Read the model definition and answer for the solid it produces. Units are mm, in the model's axes. Round coordinates to 2 decimals unless told otherwise and drop trailing zeros. Order: outer loops, then holes, each group sorted by start corner. A loop starts at its lowest first (then second) coordinate and runs counter-clockwise, first axis right, second up. Notation, with made-up numbers: (-39.75, 23.5) - (-29.75, 23.5) arc R20 cw to (-29.75, 57.5) - close; hole circle Ø8 at (18, -18). An arc over 180 degrees is marked (long way). Answer as a JSON object with one key per item and string values. Group by question number.
Q1. A cutting plane is placed at D-D on x = 41. Determine the outline of the cut face in (y, z) (3 decimals).
Q2. Given pin 1 Ø0.5 at (y, z) = (1, 1) entering from +X, flat-ended and moving along its own axis, determine where the tip first touches the part or whether it passes through.
Q3. A cutting plane is placed at C-C on x = 20.5. Determine the outline of the cut face in (y, z) (3 decimals), and give its area (3 significant figures).
Q4. Consider line 1 (X direction, y = 0.5, z = 1.8); line 2 (X direction, y = -5.5, z = 3.05); line 3 (Y direction, x = 21, z = 1.35). Determine where each line is inside the solid, lowest interval first.
Q5. A cutting plane is placed at B-B on z = 1.3. Count the separate pieces of the cut face and the enclosed holes in it, and give its area (3 significant figures).
Q6. A cutting plane is placed at A-A on y = -54.5. Determine the outline of the cut face in (x, z) (3 decimals).
Q7. The mould has two halves that part along Y. Classify faces 1 (the cylindrical face through (59.551, -59.674, 1.565)), 2 (the cylindrical face through (82.194, -74.995, 1.565)), 3 (the cylindrical face through (-24.02, 11.11, 1.57)): pulls with the +Y half, pulls with the -Y half, needs draft (parallel to the pull), parting line crosses it, or undercut.
```python
from build123d import *

# Parameters (mm, degrees)
SKETCH1_R           = 5.275384615
SKETCH1_R_2         = 3.2639
BOSS_EXTRUDE1_DEPTH = 3.175


with BuildPart() as part:
    # Sketch1 → Boss-Extrude1 (new body)
    with BuildSketch(Plane.XY):
        with BuildLine():
            Line((-14.2875, 1.5875), (-14.2875, 0))
            ThreePointArc((-14.2875, 0), (0, -14.2875), (14.2875, 0))
            Line((14.2875, 0), (14.2875, 1.5875))
            ThreePointArc((14.2875, 1.5875), (20.740075347, 10.603365557), (31.355391181, 7.403892149))
            Line((31.355391181, 7.403892149), (82.572922645, -59.016709578))
            ThreePointArc((82.572922645, -59.016709578), (82.033512438, -75.180341372), (66.05971387, -77.708525595))
            Line((66.05971387, -77.708525595), (-16.947053899, -28.708644524))
            ThreePointArc((-16.947053899, -28.708644524), (-28.951349844, -16.529012325), (-33.3375, 0))
            Line((-33.3375, 0), (-33.3375, 1.5875))
            ThreePointArc((-33.3375, 1.5875), (-23.8125, 11.1125), (-14.2875, 1.5875))
        make_face()
        with Locations((-23.8125, 0)):
            Circle(SKETCH1_R, mode=Mode.SUBTRACT)
        with Locations((23.8125, 0)):
            Circle(SKETCH1_R, mode=Mode.SUBTRACT)
        with Locations((72.515734403, -66.77189911)):
            Circle(SKETCH1_R_2, mode=Mode.SUBTRACT)
        with Locations((60.259023314, -56.487297355)):
            Circle(SKETCH1_R_2, mode=Mode.SUBTRACT)
    extrude(amount=BOSS_EXTRUDE1_DEPTH)


solid = part.part
```
Result set:
{
 "1": {"outline": "(-62.915, 0) - (-5.104, 0) - (-5.104, 3.175) - (-62.915, 3.175) - close"},
 "2": {"pin 1": "stops at x = 36.49"},
 "3": {"outline": "(-50.814, 0) - (-4.106, 0) - (-4.106, 3.175) - (-50.814, 3.175) - close; (4.106, 0) - (10.518, 0) - (10.518, 3.175) - (4.106, 3.175) - close", "area": "169 mm²"},
 "4": {"line 1": "x = -33.34 to -29.06, -18.56 to -14.29, 14.29 to 18.56, 29.06 to 36.68", "line 2": "x = -32.88 to -13.19, 13.19 to 41.31", "line 3": "y = -51.11 to -4.46, 4.46 to 10.69"},
 "5": {"separate pieces": "1", "enclosed holes": "4", "area": "4,520 mm²"},
 "6": {"outline": "(26.744, 0) - (57.67, 0) - (57.67, 3.175) - (26.744, 3.175) - close; (62.848, 0) - (79.09, 0) - (79.09, 3.175) - (62.848, 3.175) - close"},
 "7": {"face 1": "undercut", "face 2": "parting line crosses it", "face 3": "pulls with the +Y half"}
}
